```python
from build123d import *

# Parameters (mm, degrees)
SALIENTE_EXTRUIR1_DEPTH      = 10
SALIENTE_EXTRUIR1_DEPTH_BACK = 10
SALIENTE_EXTRUIR2_DEPTH      = 2
SALIENTE_EXTRUIR2_DEPTH_BACK = 2
REDONDEO1_R                  = 4
REDONDEO4_R                  = 7.3
REDONDEO2_R                  = 2
CROQUIS4_W                   = 2
CROQUIS4_H                   = 8
SALIENTE_EXTRUIR3_DEPTH      = 8
REDONDEO3_R                  = 2
CORTAR_EXTRUIR1_REACH        = 4
CROQUIS5_R                   = 2


with BuildPart() as part:
    # Croquis2 → Saliente-Extruir1 (new body, two sides)
    with BuildSketch(Plane.XY) as saliente_extruir1_sk:
        with BuildLine():
            Line((23.96097083, 4.310370238), (23.96097083, 20.310370238))
            Line((23.96097083, 20.310370238), (28.96097083, 20.310370238))
            ThreePointArc((28.96097083, 20.310370238), (35.462728392, 14.331387102), (40.877050613, 21.310370238))
            Line((40.877050613, 21.310370238), (43.877050613, 21.310370238))
            Line((43.877050613, 21.310370238), (43.877050613, 11.310370238))
            Line((43.877050613, 11.310370238), (28.96097083, 11.310370238))
            Line((28.96097083, 11.310370238), (28.96097083, 4.310370238))
            Line((28.96097083, 4.310370238), (23.96097083, 4.310370238))
        make_face()
    extrude(amount=SALIENTE_EXTRUIR1_DEPTH)
    extrude(saliente_extruir1_sk.sketch, amount=-SALIENTE_EXTRUIR1_DEPTH_BACK)

    # Croquis3 → Saliente-Extruir2 (add, two sides)
    with BuildSketch(Plane.XY) as saliente_extruir2_sk:
        Polygon((28.96097083, 4.310370238), (28.96097083, 11.310370238), (36.419010722, 11.310370238), align=None)
    extrude(amount=SALIENTE_EXTRUIR2_DEPTH)
    extrude(saliente_extruir2_sk.sketch, amount=-SALIENTE_EXTRUIR2_DEPTH_BACK)

    # Redondeo1
    redondeo1_edges = [part.edges().sort_by_distance(p)[0] for p in [
        (28.96097083, 11.310370238, -6),
        (28.96097083, 11.310370238, 6),
    ]]
    fillet(redondeo1_edges, radius=REDONDEO1_R)

    # Redondeo4
    redondeo4_edges = [part.edges().sort_by_distance(p)[0] for p in [
        (43.877050613, 11.310370238, 0),
    ]]
    fillet(redondeo4_edges, radius=REDONDEO4_R)

    # Redondeo2
    redondeo2_edges = [part.edges().sort_by_distance(p)[0] for p in [
        (28.96097083, 20.310370238, 0),
        (40.877050613, 21.310370238, 0),
    ]]
    fillet(redondeo2_edges, radius=REDONDEO2_R)

    # Croquis4 → Saliente-Extruir3 (add)
    with BuildSketch(Plane(origin=(0, 20.310370238, 0), x_dir=(1, 0, 0), z_dir=(0, 1, 0))):
        with Locations((24.96097083, 0)):
            Rectangle(CROQUIS4_W, CROQUIS4_H)
    extrude(amount=SALIENTE_EXTRUIR3_DEPTH)

    # Redondeo3
    redondeo3_edges = [part.edges().sort_by_distance(p)[0] for p in [
        (24.96097083, 20.310370238, -4),
        (24.96097083, 20.310370238, 4),
        (24.96097083, 28.310370238, -4),
        (24.96097083, 28.310370238, 4),
    ]]
    fillet(redondeo3_edges, radius=REDONDEO3_R)

    # Croquis5 → Cortar-Extruir1 (cut, up to next)
    with BuildSketch(Plane(origin=(25.96097083, 0, 0), x_dir=(0, 0, -1), z_dir=(1, 0, 0)), mode=Mode.PRIVATE) as cortar_extruir1_sk1:
        with Locations((0, 24.310370238)):
            Circle(CROQUIS5_R)
    cortar_extruir1_tool1 = extrude(cortar_extruir1_sk1.sketch, amount=-CORTAR_EXTRUIR1_REACH, mode=Mode.PRIVATE) & part.part
    add(cortar_extruir1_tool1.solids().sort_by_distance((25.960971, 24.31037, 0))[0], mode=Mode.SUBTRACT)


solid = part.part
```
Could you check a few things on this model? Use its own coordinates, in mm. A direction names the side the tool comes from. Coordinates: 2 decimals unless noted, no trailing zeros. Write each loop counter-clockwise with the first axis right and the second up, starting at its lowest first coordinate (ties: lowest second). Pieces come first, ordered by that corner, then holes. Notation, with made-up numbers: (24.25, 34) - (82.25, 34) arc R14 ccw to (82.25, 52) - close; hole circle Ø9 at (55, 45). An arc over 180 degrees is marked (long way). Use a Markdown table: item, result.
Q1. Please list where these lines run through material, in increasing order: L1, parallel to Y at x = 25.4, z = 0; L2, parallel to Y at x = 27, z = -5.25; L3, parallel to Z at x = 30.75, y = 7.5.
Geometry check:
| item | result |
|---|---|
| L1 | y = 4.31 to 22.31, 26.31 to 28.31 |
| L2 | y = 4.31 to 20.31 |
| L3 | z = -2 to 2 |
Q2. Thinking about a two-plate mould opening in X: for faces 6 (the flat face through (32, 13, -10)), 7 (the cylindrical face through (35.227, 14.316, 0.14)), 8 (the cylindrical face through (30, 10, 6)), 9 (the flat face through (23.961, 13, 0)), which applies, +X half, -X half, draft (parallel to the pull), parting line (faces both ways), or undercut?
Geometry check:
| item | result |
|---|---|
| face 6 | draft |
| face 7 | undercut |
| face 8 | +X half |
| face 9 | -X half |
Q3. I'm going to push flat-ended pins straight in: pin 1 Ø3.5 at (y, z) = (6, -5.5) entering from +X; pin 2 Ø1 at (x, z) = (36.5, -3.5) entering from -Y; pin 3 Ø1.8 at (x, z) = (34, 2.5) entering from -Y. Where does each tip first touch, or does it pass through?
Geometry check:
| item | result |
|---|---|
| pin 1 | stops at x = 28.99 |
| pin 2 | stops at y = 11.31 |
| pin 3 | stops at y = 8.34 |
Q4. Imagine slicing it at B-B (y = 19.25). List the corners of the cut face in (x, z) for me.
Geometry check:
| item | result |
|---|---|
| outline | (23.96, -10) - (28.98, -10) - (28.98, 10) - (23.96, 10) - close; (40.87, -10) - (43.88, -10) - (43.88, 10) - (40.87, 10) - close |
Q5. Imagine slicing it at D-D (z = -6.75). List the corners of the cut face in (x, y) for me (1 decimal), and give its area (3 significant figures).
Geometry check:
| item | result |
|---|---|
| outline | (24, 4.3) - (29, 4.3) - (29, 7.3) arc R4 cw to (33, 11.3) - (36.6, 11.3) arc R7.3 ccw to (43.9, 18.6) - (43.9, 21.3) - (42.9, 21.3) arc R2 ccw to (40.9, 19.6) arc R6 cw to (29.2, 18.8) arc R2 ccw to (27.2, 20.3) - (24, 20.3) - close |
| area | 151 mm2 |
Q6. Imagine slicing it at C-C (x = 34.75). List the corners of the cut face in (y, z) for me, and give its area (3 significant figures).
Geometry check:
| item | result |
|---|---|
| outline | (9.74, -2) - (11.31, -2) - (11.31, -10) - (14.31, -10) - (14.31, 10) - (11.31, 10) - (11.31, 2) - (9.74, 2) - close |
| area | 66.3 mm2 |
Q7. Which directions (+Z, -Z, +X, -X, +Y, -Y) give clear straight access to the entire face, cutting with the end or side of a thin tool? Please do faces 1 (the flat face through (43.4, 21.31, 0.1)), 2 (the flat face through (34.8, 11.31, 2.4)), 3 (the cylindrical face through (41.591, 20.824, -0.14)), 4 (the cylindrical face through (24.97, 20.88, 4.6)), 5 (the flat face through (28.961, 6, -6)).
Geometry check:
| item | result |
|---|---|
| face 1 | +Z, -Z, +X, +Y |
| face 2 | +X, -Y |
| face 3 | +Z, -Z, +Y |
| face 4 | +Z, -X, +Y |
| face 5 | -Z, +X, -Y |
